from build123d import *

# Parameters (mm, degrees)
F0_R     = 3
F1_DEPTH = 1.2
F2_R     = 3
F2_W     = 43.6
F2_H     = 43.6
F3_DEPTH = 6.4
F4_R     = 3
F4_W     = 46
F4_H     = 46
F5_DEPTH = 1.6
F6_R     = 3
F7_DEPTH = 3
F9_DEPTH = 3.2
F10_R    = 0.99999
F11_R    = 3


# Not quite as in the source:
# - a fillet or chamfer is up to 0.001 mm smaller than in the source, because OpenCascade refuses the exact size


with BuildPart() as f1:
    # F0 (on Top) → F1 (new body)
    with BuildSketch(Plane.XY):
        with BuildLine():
            Line((22.8786796564, 31.3639610307), (16.5147186258, 25))
            Line((16.5147186258, 25), (-25, 25))
            Line((-25, 25), (-25, -16.5147186258))
            Line((-25, -16.5147186258), (-31.3639610307, -22.8786796564))
            ThreePointArc((-31.3639610307, -22.8786796564), (-31.3639610307, -31.3639610307), (-22.8786796564, -31.3639610307))
            Line((-22.8786796564, -31.3639610307), (-16.5147186258, -25))
            Line((-16.5147186258, -25), (25, -25))
            Line((25, -25), (25, 16.5147186258))
            Line((25, 16.5147186258), (31.3639610307, 22.8786796564))
            ThreePointArc((31.3639610307, 22.8786796564), (31.3639610307, 31.3639610307), (22.8786796564, 31.3639610307))
        make_face()
        with Locations((-27.1213203436, -27.1213203436)):
            Circle(F0_R, mode=Mode.SUBTRACT)
        with Locations((27.1213203436, 27.1213203436)):
            Circle(F0_R, mode=Mode.SUBTRACT)
    extrude(amount=F1_DEPTH)

    # F2 (on face) → F3 (join)
    with BuildSketch(Plane.XY.offset(1.2)):
        with BuildLine():
            Line((-16.5147186258, -25), (25, -25))
            Line((25, -25), (25, 16.5147186258))
            Line((25, 16.5147186258), (31.3639610307, 22.8786796564))
            ThreePointArc((31.3639610307, 22.8786796564), (31.3639610307, 31.3639610307), (22.8786796564, 31.3639610307))
            Line((22.8786796564, 31.3639610307), (16.5147186258, 25))
            Line((16.5147186258, 25), (-25, 25))
            Line((-25, 25), (-25, -16.5147186258))
            Line((-25, -16.5147186258), (-31.3639610307, -22.8786796564))
            ThreePointArc((-31.3639610307, -22.8786796564), (-31.3639610307, -31.3639610307), (-22.8786796564, -31.3639610307))
            Line((-22.8786796564, -31.3639610307), (-16.5147186258, -25))
        make_face()
        with Locations((-27.1213203436, -27.1213203436)):
            Circle(F2_R, mode=Mode.SUBTRACT)
        Rectangle(F2_W, F2_H, mode=Mode.SUBTRACT)
        with Locations((27.1213203436, 27.1213203436)):
            Circle(F2_R, mode=Mode.SUBTRACT)
    extrude(amount=F3_DEPTH)

    # F4 (on face) → F5 (join)
    with BuildSketch(Plane.XY.offset(7.6)):
        with BuildLine():
            Line((-16.5147186258, -25), (25, -25))
            Line((25, -25), (25, 16.5147186258))
            Line((25, 16.5147186258), (31.3639610307, 22.8786796564))
            ThreePointArc((31.3639610307, 22.8786796564), (31.3639610307, 31.3639610307), (22.8786796564, 31.3639610307))
            Line((22.8786796564, 31.3639610307), (16.5147186258, 25))
            Line((16.5147186258, 25), (-25, 25))
            Line((-25, 25), (-25, -16.5147186258))
            Line((-25, -16.5147186258), (-31.3639610307, -22.8786796564))
            ThreePointArc((-31.3639610307, -22.8786796564), (-31.3639610307, -31.3639610307), (-22.8786796564, -31.3639610307))
            Line((-22.8786796564, -31.3639610307), (-16.5147186258, -25))
        make_face()
        with Locations((-27.1213203436, -27.1213203436)):
            Circle(F4_R, mode=Mode.SUBTRACT)
        Rectangle(F4_W, F4_H, mode=Mode.SUBTRACT)
        with Locations((27.1213203436, 27.1213203436)):
            Circle(F4_R, mode=Mode.SUBTRACT)
    extrude(amount=F5_DEPTH)

    # F6 (on face) → F7 (join)
    with BuildSketch(Plane.XY.offset(9.2)):
        Polygon((15, -25), (25, -25), (25, -15), (23, -15), (23, -23), (15, -23), align=None)
        with BuildLine():
            Line((25, 15), (25, 16.5147186258))
            Line((25, 16.5147186258), (31.3639610307, 22.8786796564))
            ThreePointArc((31.3639610307, 22.8786796564), (31.3639610307, 31.3639610307), (22.8786796564, 31.3639610307))
            Line((22.8786796564, 31.3639610307), (16.5147186258, 25))
            Line((16.5147186258, 25), (15, 25))
            Line((15, 25), (15, 23))
            Line((15, 23), (23, 23))
            Line((23, 23), (23, 15))
            Line((23, 15), (25, 15))
        make_face()
        with Locations((27.1213203436, 27.1213203436)):
            Circle(F6_R, mode=Mode.SUBTRACT)
        Polygon((-15, 25), (-25, 25), (-25, 15), (-23, 15), (-23, 23), (-15, 23), align=None)
        with BuildLine():
            Line((-25, -15), (-25, -16.5147186258))
            Line((-25, -16.5147186258), (-31.3639610307, -22.8786796564))
            ThreePointArc((-31.3639610307, -22.8786796564), (-31.3639610307, -31.3639610307), (-22.8786796564, -31.3639610307))
            Line((-22.8786796564, -31.3639610307), (-16.5147186258, -25))
            Line((-16.5147186258, -25), (-15, -25))
            Line((-15, -25), (-15, -23))
            Line((-15, -23), (-23, -23))
            Line((-23, -23), (-23, -15))
            Line((-23, -15), (-25, -15))
        make_face()
        with Locations((-27.1213203436, -27.1213203436)):
            Circle(F6_R, mode=Mode.SUBTRACT)
    extrude(amount=F7_DEPTH)

    # F8 (on face) → F9 (cut, through all)
    with BuildSketch(Plane(origin=(0, 25, 0), x_dir=(-1, 0, 0), z_dir=(0, 1, 0))):
        with BuildLine():
            Line((-3.2, 9.2), (-3.2, 4.4))
            ThreePointArc((-3.2, 4.4), (0, 1.2), (3.2, 4.4))
            Line((3.2, 4.4), (3.2, 9.2))
            Line((3.2, 9.2), (-3.2, 9.2))
        make_face()
    extrude(amount=-F9_DEPTH, mode=Mode.SUBTRACT)

    # F10 (radius 1 in the source; OpenCascade refuses exactly that, so slightly less here)
    f10_edges = [f1.edges().sort_by_distance(p)[0] for p in [
        (25, -15, 10.7),
        (23, -15, 10.7),
        (15, -25, 10.7),
        (15, -23, 10.7),
        (-15, -25, 10.7),
        (-15, -23, 10.7),
        (-23, -15, 10.7),
        (-23, 15, 10.7),
        (-25, -15, 10.7),
        (-15, 23, 10.7),
        (-15, 25, 10.7),
        (15, 23, 10.7),
        (15, 25, 10.7),
        (23, 15, 10.7),
        (25, 15, 10.7),
    ]]
    fillet(f10_edges, radius=F10_R)

    # F11
    f11_edges = [f1.edges().sort_by_distance(p)[0] for p in [
        (-25, 25, 6.1),
        (25, -25, 6.1),
    ]]
    fillet(f11_edges, radius=F11_R)


solid = f1.part
CAD build for the part. Positions are in the model's coordinates, mm. A direction names the side the tool comes from. Coordinates: 2 decimals unless noted, no trailing zeros. Loops run counter-clockwise (first coordinate to the right, second up) from the corner with the lowest first, then second, coordinate; pieces in that order, holes last. Notation, with made-up numbers: (4.5, 79.25) - (31.5, 79.25) arc R23 cw to (31.5, 104.25) - close; hole circle Ø6 at (-16.5, 48.25). An arc over 180 degrees is marked (long way). Write item = value, one per line. Start each with the question number.
Q1. Cut at C-C, the plane y = 11. List the corners of the cut face in (x, z).
Q2. Flat gauge pins, fed straight in: pin 1 Ø0.6 at (x, y) = (11, 24) entering from +Z; pin 2 Ø1.5 at (y, z) = (4.5, 6.5) entering from +X; pin 3 Ø3.5 at (x, z) = (-4, 3.5) entering from -Y; pin 4 Ø2 at (x, z) = (-9.5, 11) entering from -Y. Where does each tip first touch, or does it go through?
Q3. Drill centre lines: L1, parallel to X at y = 6, z = 2.25; L2, parallel to Z at x = -14, y = 2.5. Where is each one in solid material? Low to high.
Q4. Which spindle directions (+Z, -Z, +X, -X, +Y, -Y) get a long thin tool onto all of the face, cutting with end or side? Do faces 4 (the flat face through (-28.137, -19.652, 6.015)), 5 (the flat face through (-23, 0, 9)). Say none if no direction does.
Q5. Cut at A-A, the plane x = 29. List the corners of the cut face in (y, z), then the cut area to 4 significant figures.
Q6. Cut at B-B, the plane z = 5.25. List the corners of the cut face in (x, y), then the cut area to 3 significant figures.
Q7. Pull direction X, two halves, no side cores. Call faces 1 (the flat face through (23, 0, 9)), 2 (the flat face through (0, 0, 0)), 3 (the flat face through (28.137, 19.652, 6.015)): pulls with the +X half, pulls with the -X half, needs draft (parallel to the pull), parting line crosses it, or undercut.
Computed:
q1.outline = (-25, 0) - (25, 0) - (25, 9.2) - (23, 9.2) - (23, 7.6) - (21.8, 7.6) - (21.8, 1.2) - (-21.8, 1.2) - (-21.8, 7.6) - (-23, 7.6) - (-23, 9.2) - (-25, 9.2) - close
q2.pin_1 = 9.2
q2.pin_2 = 25
q2.pin_3 = -25
q2.pin_4 = through
q3.L1 = -25 to -21.8, 21.8 to 25
q3.L2 = 0 to 1.2
q4.face_4 = +Z, -Z, -X, +Y
q4.face_5 = +Z
q5.outline = (20.51, 0) - (24.78, 0) - (24.78, 12.2) - (20.51, 12.2) - close; (29.46, 0) - (32.82, 0) - (32.82, 12.2) - (29.46, 12.2) - close
q5.area = 93.05 mm²
q6.outline = (-31.36, -22.88) arc R6 ccw to (-22.88, -31.36) - (-16.51, -25) - (22, -25) arc R3 ccw to (25, -22) - (25, 16.51) - (31.36, 22.88) arc R6 ccw to (22.88, 31.36) - (16.51, 25) - (3.2, 25) - (3.2, 21.8) - (21.8, 21.8) - (21.8, -21.8) - (-21.8, -21.8) - (-21.8, 21.8) - (-3.2, 21.8) - (-3.2, 25) - (-22, 25) arc R3 ccw to (-25, 22) - (-25, -16.51) - close; hole circle Ø6 at (-27.12, -27.12); hole circle Ø6 at (27.12, 27.12)
q6.area = 775 mm²
q7.face_1 = undercut
q7.face_2 = needs draft
q7.face_3 = pulls with the +X half
